The model under review builds one solid part; all positions refer to its coordinate system, in mm. Face numbers are marked on the shaded views. A direction names the side the tool comes from. Round coordinates to 2 decimals unless told otherwise and drop trailing zeros. Loops run counter-clockwise (first coordinate to the right, second up) from the corner with the lowest first, then second, coordinate; pieces in that order, holes last. Notation, with made-up numbers: M -22.75,22.25 L 5.25,22.25 A8 ccw 5.25,30.25 Z; hole C -3.75,-22 d2. An arc over 180 degrees is marked long. Answer as a JSON object with one key per item and string values. Group by question number.
Item 1: Consider section C-C (x = 0). Give the boundary of the cut face in (y, z), and give its area (3 significant figures).
Item 2: Consider section A-A (y = 83). Give the boundary of the cut face in (x, z), and give its area (3 significant figures).
Item 3: Consider section D-D (z = 16.5). State how many separate pieces and enclosed holes the cut face has, and give its area (3 significant figures).
Item 4: To check wall thickness, follow line 1 (X direction, y = 1, z = -23.5); line 2 (Z direction, x = 0, y = 104); line 3 (X direction, y = 88, z = 14). State the ranges of each line that lie inside material, in increasing order.
Item 5: Consider section B-B (y = 64). Give the boundary of the cut face in (x, z), and give its area (3 significant figures).
Item 6: Insertion check: P1, Ø4, axis at y = -0.5, z = -3, coming from the +X side; P2, Ø2, axis at y = 82.5, z = -7, coming from the -X side; P3, Ø6, axis at x = 38.5, y = 42.5, coming from the +Z side; P4, Ø4, axis at x = -0.5, z = 21, coming from the -Y side. Each pin has a flat end and moves straight along its axis. Give the tip position at first contact, or say it passes through.
Item 7: Tool access review of the marked faces 1, 2 and 3: name each direction out of +Z, -Z, +X, -X, +Y, -Y from which nothing blocks a thin tool from reaching the whole face with its end or side.
Item 8: The part is to be moulded in two halves that separate along Y. For the marked faces 4, 5 and 6, say which applies: +Y half, -Y half, draft (parallel to the pull), parting line (faces both ways), or undercut.
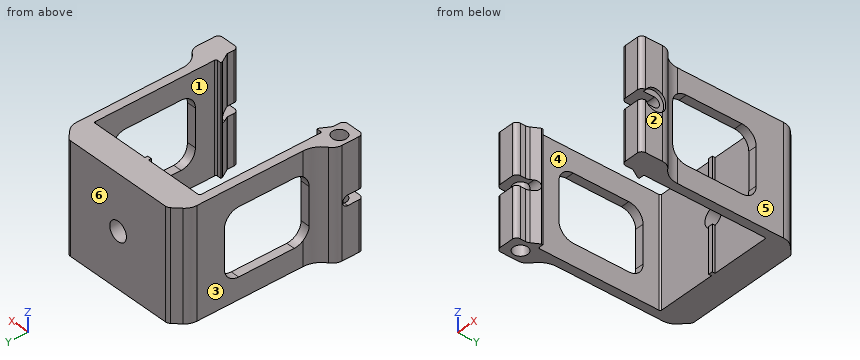
```python
from build123d import *

# Parameters (mm, degrees)
BOSS_EXTRUDE1_DEPTH     = 38.1
SKETCH4_R               = 5
CUT_EXTRUDE2_DEPTH      = 147.798126691
FILLET1_R               = 1
FILLET2_R               = 4
BOSS_EXTRUDE5_START     = -76.2
BOSS_EXTRUDE5_DEPTH     = 76.2
SKETCH9_R               = 7.5
CUT_EXTRUDE3_DEPTH      = 2
SKETCH10_W              = 3
SKETCH10_H              = 76.2
BOSS_EXTRUDE4_DEPTH     = 2
CUT_EXTRUDE1_DEPTH      = 166.715448911
CUT_EXTRUDE8_DEPTH      = 166.715448911
CUT_EXTRUDE10_DEPTH     = 147.798126783
F_5_8_11_TAPPED_HOLE1_D = 13.49248
FILLET3_R               = 10


with BuildPart() as part:
    # Sketch1 → Boss-Extrude1 (new, symmetric)
    with BuildSketch(Plane.XY):
        with BuildLine():
            Line((-42.75, 91), (42.75, 91))
            Line((42.75, 91), (42.75, 6.5))
            ThreePointArc((42.75, 6.5), (42.457106781, 5.792893219), (41.75, 5.5))
            Line((41.75, 5.5), (38.933657049, 5.5))
            Line((38.933657049, 5.5), (38.933657049, 4.5))
            Line((38.933657049, 4.5), (42.616025404, -1.878049083))
            ThreePointArc((42.616025404, -1.878049083), (42.715925826, -2.119230038), (42.75, -2.378049083))
            Line((42.75, -2.378049083), (42.75, -7))
            ThreePointArc((42.75, -7), (43.628679656, -9.121320344), (45.75, -10))
            Line((45.75, -10), (55.5, -10))
            ThreePointArc((55.5, -10), (57.621320344, -9.121320344), (58.5, -7))
            Line((58.5, -7), (58.5, 92.5))
            Line((58.5, 92.5), (40, 111))
            Line((40, 111), (-40, 111))
            Line((-40, 111), (-58.5, 92.5))
            Line((-58.5, 92.5), (-58.5, 0))
            ThreePointArc((-58.5, 0), (-52.66319998, -7.606665882), (-43.805049945, -3.9375))
            Line((-43.805049945, -3.9375), (-38.933657049, 4.5))
            Line((-38.933657049, 4.5), (-38.933657049, 5.5))
            Line((-38.933657049, 5.5), (-41.75, 5.5))
            ThreePointArc((-41.75, 5.5), (-42.457106781, 5.792893219), (-42.75, 6.5))
            Line((-42.75, 6.5), (-42.75, 91))
        make_face()
    extrude(amount=BOSS_EXTRUDE1_DEPTH, both=True)

    # Sketch4 → Cut-Extrude2 (cut, through all)
    with BuildSketch(Plane.XY.offset(38.1)):
        with Locations((-50.625, 0)):
            Circle(SKETCH4_R)
    extrude(amount=-CUT_EXTRUDE2_DEPTH, mode=Mode.SUBTRACT)

    # Fillet1
    fillet1_edges = [part.edges().sort_by_distance(p)[0] for p in [
        (42.75, 91, 0),
        (-42.75, 91, 0),
    ]]
    fillet(fillet1_edges, radius=FILLET1_R)

    # Fillet2
    fillet2_edges = [part.edges().sort_by_distance(p)[0] for p in [
        (-58.5, 92.5, 0),
        (-40, 111, 0),
        (40, 111, 0),
        (58.5, 92.5, 0),
    ]]
    fillet(fillet2_edges, radius=FILLET2_R)

    # Sketch14 → Boss-Extrude5 (add)
    with BuildSketch(Plane(origin=(0, 0, -38.1), x_dir=(-1, 0, 0), z_dir=(0, 0, -1)).offset(BOSS_EXTRUDE5_START)):
        with BuildLine():
            Line((45.75, -10), (55.5, -10))
            ThreePointArc((55.5, -10), (57.621320344, -9.121320344), (58.5, -7))
            Line((58.5, -7), (58.5, 0))
            ThreePointArc((58.5, 0), (52.66319998, -7.606665882), (43.805049945, -3.9375))
            Line((43.805049945, -3.9375), (42.080127019, -0.949845853))
            ThreePointArc((42.080127019, -0.949845853), (42.579629131, -2.155750627), (42.75, -3.449845853))
            Line((42.75, -3.449845853), (42.75, -7))
            ThreePointArc((42.75, -7), (43.628679656, -9.121320344), (45.75, -10))
        make_face()
    extrude(amount=BOSS_EXTRUDE5_DEPTH)

    # Sketch9 → Cut-Extrude3 (cut)
    with BuildSketch(Plane(origin=(58.5, 0, 0), x_dir=(0, 0, -1), z_dir=(1, 0, 0))):
        with Locations(Location((0, 0, 0), (0, 0, 90))):
            Circle(SKETCH9_R)
    extrude(amount=-CUT_EXTRUDE3_DEPTH, mode=Mode.SUBTRACT)

    # Sketch10 → Boss-Extrude4 (add)
    with BuildSketch(Plane.XZ.offset(-91)):
        Rectangle(SKETCH10_W, SKETCH10_H)
    extrude(amount=BOSS_EXTRUDE4_DEPTH)

    # Sketch3 → Cut-Extrude1 (cut, through all)
    with BuildSketch(Plane(origin=(58.5, 0, 0), x_dir=(0, 0, -1), z_dir=(1, 0, 0))):
        with BuildLine():
            Line((3.5, 1), (3.5, -10))
            ThreePointArc((3.5, -10), (0, -13.5), (-3.5, -10))
            Line((-3.5, -10), (-3.5, 1))
            ThreePointArc((-3.5, 1), (0, 4.5), (3.5, 1))
        make_face()
    extrude(amount=-CUT_EXTRUDE1_DEPTH, mode=Mode.SUBTRACT)

    # Sketch18 → Cut-Extrude8 (cut, through all)
    with BuildSketch(Plane.ZY.offset(58.5)):
        with BuildLine():
            Line((-13.1, 78.843145751), (13.1, 78.843145751))
            ThreePointArc((13.1, 78.843145751), (20.171067812, 75.914213562), (23.1, 68.843145751))
            Line((23.1, 68.843145751), (23.1, 30))
            ThreePointArc((23.1, 30), (20.171067812, 22.928932188), (13.1, 20))
            Line((13.1, 20), (-13.1, 20))
            ThreePointArc((-13.1, 20), (-20.171067812, 22.928932188), (-23.1, 30))
            Line((-23.1, 30), (-23.1, 68.843145751))
            ThreePointArc((-23.1, 68.843145751), (-20.171067812, 75.914213562), (-13.1, 78.843145751))
        make_face()
    extrude(amount=-CUT_EXTRUDE8_DEPTH, mode=Mode.SUBTRACT)

    # Sketch22 → Cut-Extrude10 (cut, through all)
    with BuildSketch(Plane(origin=(0, 0, -38.1), x_dir=(-1, 0, 0), z_dir=(0, 0, -1))):
        with BuildLine():
            Line((48.75, 102.25), (48.75, 23.799933511))
            ThreePointArc((48.75, 23.799933511), (50.434228051, 16.894123103), (55.108695652, 11.539107308))
            ThreePointArc((55.108695652, 11.539107308), (57.60174504, 8.683098884), (58.5, 5))
            Line((58.5, 5), (58.5, 90.843145751))
            ThreePointArc((58.5, 90.843145751), (58.19551813, 92.37387948), (57.328427125, 93.671572875))
            Line((57.328427125, 93.671572875), (48.75, 102.25))
        make_face()
        with BuildLine():
            Line((-48.75, 23.799933511), (-48.75, 102.25))
            Line((-48.75, 102.25), (-57.328427125, 93.671572875))
            ThreePointArc((-57.328427125, 93.671572875), (-58.19551813, 92.37387948), (-58.5, 90.843145751))
            Line((-58.5, 90.843145751), (-58.5, 5))
            ThreePointArc((-58.5, 5), (-57.60174504, 8.683098884), (-55.108695652, 11.539107308))
            ThreePointArc((-55.108695652, 11.539107308), (-50.434228051, 16.894123103), (-48.75, 23.799933511))
        make_face()
    extrude(amount=-CUT_EXTRUDE10_DEPTH, mode=Mode.SUBTRACT)

    # 5/8-11 Tapped Hole1 (through all)
    with Locations(Plane(origin=(0, 111, 0), x_dir=(1, 0, 0), z_dir=(0, 1, 0))):
        with Locations((0, 0)):
            Hole(F_5_8_11_TAPPED_HOLE1_D / 2)

    # Fillet3
    fillet3_edges = [part.edges().sort_by_distance(p)[0] for p in [
        (-48.75, 102.25, 0),
        (48.75, 102.25, 0),
    ]]
    fillet(fillet3_edges, radius=FILLET3_R)


solid = part.part
```
Geometry results:
{
 "1": {"outline": "M 89,-38.1 L 111,-38.1 L 111,-6.75 L 89,-6.75 Z; M 89,6.75 L 111,6.75 L 111,38.1 L 89,38.1 Z", "area": "1,380 mm^2"},
 "2": {"outline": "M -48.75,-38.1 L -42.75,-38.1 L -42.75,38.1 L -48.75,38.1 Z; M 42.75,-38.1 L 48.75,-38.1 L 48.75,38.1 L 42.75,38.1 Z", "area": "914 mm^2"},
 "3": {"separate pieces": "3", "enclosed holes": "1", "area": "2,790 mm^2"},
 "4": {"line 1": "x = -58.5 to -55.52, -45.73 to -40.95, 40.95 to 58.5", "line 2": "z = -38.1 to -6.75, 6.75 to 38.1", "line 3": "x = -48.75 to -42.75, 42.75 to 48.75"},
 "5": {"outline": "M -48.75,-38.1 L -42.75,-38.1 L -42.75,-23.1 L -48.75,-23.1 Z; M -48.75,23.1 L -42.75,23.1 L -42.75,38.1 L -48.75,38.1 Z; M 42.75,-38.1 L 48.75,-38.1 L 48.75,-23.1 L 42.75,-23.1 Z; M 42.75,23.1 L 48.75,23.1 L 48.75,38.1 L 42.75,38.1 Z", "area": "360 mm^2"},
 "6": {"P1": "stops at x = 56.5", "P2": "stops at x = -48.75", "P3": "passes through", "P4": "stops at y = 89"},
 "7": {"face 1": "+Z, -Z", "face 2": "+Z, -Z, +X, +Y, -Y", "face 3": "+Z, -Z, -X, +Y"},
 "8": {"face 4": "undercut", "face 5": "draft", "face 6": "+Y half"}
}
